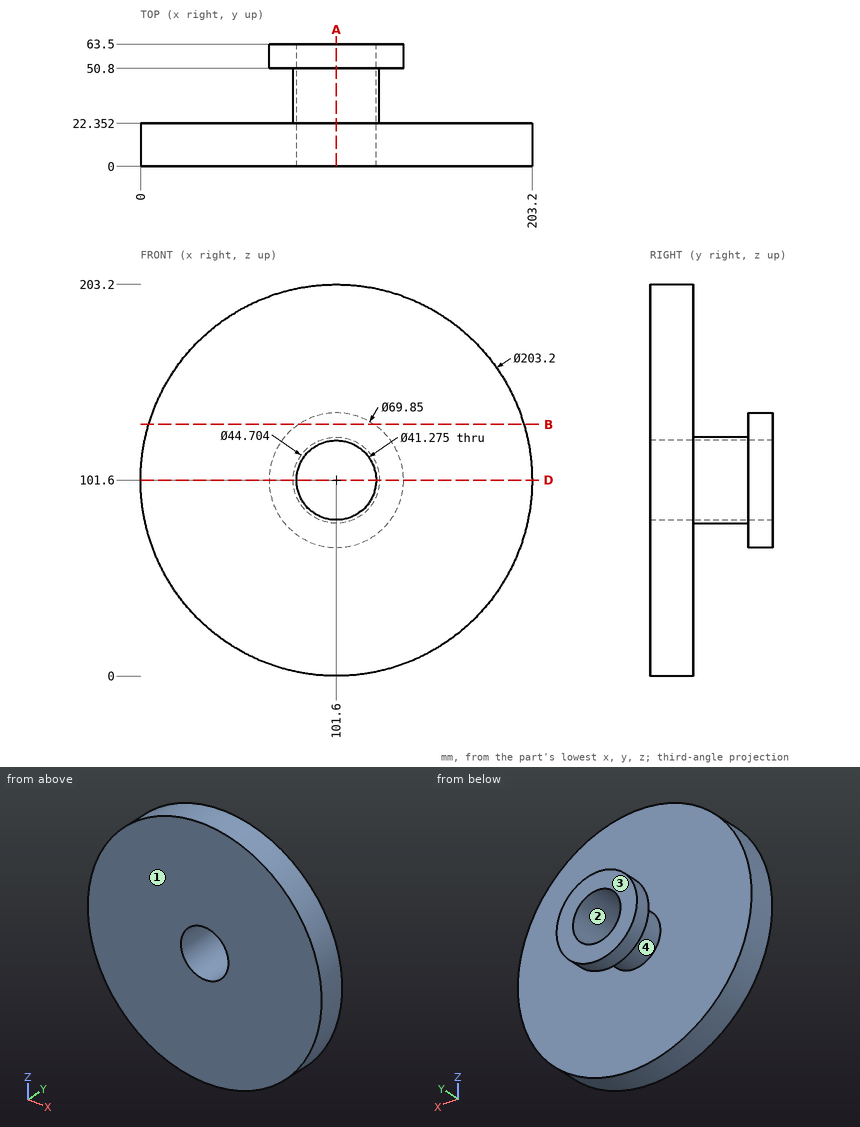
Can you work these out from the drawing? Everything is in mm from the part's minimum corner. Give positions to 0.01 mm unless a question says otherwise; leave off trailing zeros. Write each loop counter-clockwise with the first axis right and the second up, starting at its lowest first coordinate (ties: lowest second). Pieces come first, ordered by that corner, then holes. Notation, with made-up numbers: (81.25, 2) -> (112.25, 2) arc R29 cw to (112.25, 28) -> close; hole circle Ø8 at (32, 23.25). An arc over 180 degrees is marked (long way). Write each question's results on one line, items separated by ' | '.
Item 1: Suppose I cut it at A-A on x = 101.6. Write out the boundary of the cut face in (y, z) (1 decimal).
Output:
outline: (0, 0) -> (22.4, 0) -> (22.4, 79.2) -> (50.8, 79.2) -> (50.8, 66.7) -> (63.5, 66.7) -> (63.5, 81) -> (0, 81) -> close; (0, 122.2) -> (63.5, 122.2) -> (63.5, 136.5) -> (50.8, 136.5) -> (50.8, 124) -> (22.4, 124) -> (22.4, 203.2) -> (0, 203.2) -> close
Item 2: Suppose I cut it at D-D on z = 101.6. Write out the boundary of the cut face in (x, y) (1 decimal).
Output:
outline: (0, 0) -> (81, 0) -> (81, 63.5) -> (66.7, 63.5) -> (66.7, 50.8) -> (79.2, 50.8) -> (79.2, 22.4) -> (0, 22.4) -> close; (122.2, 0) -> (203.2, 0) -> (203.2, 22.4) -> (124, 22.4) -> (124, 50.8) -> (136.5, 50.8) -> (136.5, 63.5) -> (122.2, 63.5) -> close
Item 3: Suppose I cut it at B-B on z = 130.5. Write out the boundary of the cut face in (x, y).
Output:
outline: (4.2, 0) -> (199, 0) -> (199, 22.35) -> (4.2, 22.35) -> close; (81.99, 50.8) -> (121.21, 50.8) -> (121.21, 63.5) -> (81.99, 63.5) -> close
Item 4: We'd pull the mould along Y, two halves only. Please class the marked faces 1, 2, 3 and 4: pulls with the +Y half, pulls with the -Y half, needs draft (parallel to the pull), parting line crosses it, or undercut.
Output:
face 1: pulls with the -Y half | face 2: needs draft | face 3: pulls with the +Y half | face 4: undercut
Item 5: If I drill on L1, parallel to Y at x = 124, z = 113; L2, parallel to X at y = 19, z = 101.6; L3, parallel to Y at x = 43, z = 25.5, over which ranges is the centre line in solid material (lowest first)?
Output:
L1: y = 0 to 22.35, 50.8 to 63.5 | L2: x = 0 to 80.96, 122.24 to 203.2 | L3: y = 0 to 22.35
Item 6: For pin 1 Ø4 at (x, y) = (151, 13.5) entering from -Z; pin 2 Ø10 at (x, z) = (36, 49.5) entering from +Y; pin 3 Ø1.5 at (y, z) = (55, 68.5) entering from +X, each with a flat end and sliding along its axis, tell me the tip position at first contact or that it passes through.
Output:
pin 1: stops at z = 11.73 | pin 2: stops at y = 22.35 | pin 3: stops at x = 114.76
